Verification items for the finished model (mm, model axes). Face numbers are marked on the shaded views. A direction names the side the tool comes from. Give positions to 0.01 mm unless a question says otherwise; leave off trailing zeros. Order: outer loops, then holes, each group sorted by start corner. A loop starts at its lowest first (then second) coordinate and runs counter-clockwise, first axis right, second up.
(1) Sectioned sample at B-B on y = 8. Record the cut outline in (x, z).
(2) Sectioned sample at D-D on x = 9.25. Record the cut outline in (y, z).
(3) Access from +Z, -Z, +X, -X, +Y, -Y to the whole of each face (thin tool, end or side, straight path). Record for the marked faces 1 and 2.
(4) Scan lines: L1, parallel to Y at x = -10.5, z = 3.25; L2, parallel to Y at x = -1, z = 2; L3, parallel to Y at x = -4.25, z = 4.75. Record each from-to range of solid material in increasing order.
(5) Gauge pin test, flat ends, axial feed: pin 1 (4 mm diameter, centred on x = -2, z = 3.5, fed in from +Y); pin 2 (6 mm diameter, centred on x = -1.5, z = 9, fed in from +Y); pin 3 (10 mm diameter, centred on x = 3, y = 43.5, fed in from +Z). Record the tip position at first contact, or that the pin passes through.
(6) Sectioned sample at C-C on x = -4.5. Record the cut outline in (y, z).
(7) Sectioned sample at A-A on x = 0. Record the cut outline in (y, z).
```python
from build123d import *

# Parameters (mm, degrees)
SKETCH1_R           = 8
BOSS_EXTRUDE1_DEPTH = 25
SKETCH2_R           = 12.5
BOSS_EXTRUDE2_DEPTH = 5
SKETCH4_R           = 2.5


with BuildPart() as part:
    # Sketch1 → Boss-Extrude1 (new body)
    with BuildSketch(Plane(origin=(0, 0, 0), x_dir=(1, 0, 0), z_dir=(0, 1, 0))):
        with Locations(Location((0, 0, 0), (0, 0, 270))):
            Circle(SKETCH1_R)
    extrude(amount=BOSS_EXTRUDE1_DEPTH)

    # Sketch2 → Boss-Extrude2 (add)
    with BuildSketch(Plane(origin=(0, 25, 0), x_dir=(1, 0, 0), z_dir=(0, 1, 0))):
        with Locations(Location((0, 0, 0), (0, 0, 270))):
            Circle(SKETCH2_R)
    extrude(amount=BOSS_EXTRUDE2_DEPTH)

    # Sweep1: sweep along a path in Sketch3
    with BuildLine(Plane(origin=(0, 0, 0), x_dir=(0, 0, -1), z_dir=(1, 0, 0))) as sweep1_path:
        ThreePointArc((4.961180913, 27.822787702), (-0.153256004, 46.504163807), (-4.692751062, 27.67481802))
    # Sketch4 → Sweep1 (sweep)
    with BuildSketch(Plane.XY):
        with Locations((0, 46.505338246)):
            Circle(SKETCH4_R)
    sweep(path=sweep1_path.line)


solid = part.part
```
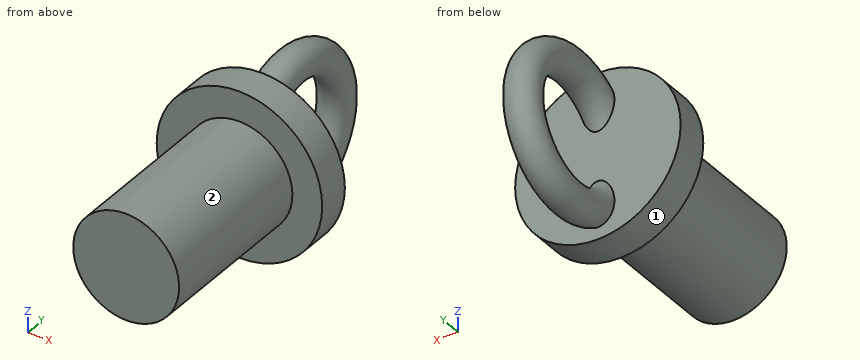
Ans:
1. outline: circle Ø16 at (0, 0)
2. outline: (25, -8.41) - (30, -8.41) - (30, 8.41) - (25, 8.41) - close
3. face 1: +Y, -Y
3. face 2: -Y
4. L1: y = 25 to 30
4. L2: y = 0 to 30, 43.95 to 48.63
4. L3: y = 0 to 30
5. pin 1: stops at y = 48.76
5. pin 2: stops at y = 47.32
5. pin 3: stops at z = 12.17
6. outline: (0, -6.61) - (25, -6.61) - (25, -11.66) - (30, -11.66) - (30, 11.66) - (25, 11.66) - (25, 6.61) - (0, 6.61) - close
7. outline: (0, -8) - (25, -8) - (25, -12.5) - (30, -12.5) - (30, -10.67) arc R12.5 ccw (long way) to (30, 10.67) - (30, 12.5) - (25, 12.5) - (25, 8) - (0, 8) - close; hole (30, -3.73) arc R7.5 ccw (long way) to (30, 3.73) - close
